```python
from build123d import *

# Parameters (mm, degrees)
BOSS_EXTRUDE1_DEPTH  = 10
M3_CLEARANCE_HOLE1_D = 3.4
FILLET1_R            = 1.5
FILLET2_R            = 0.5


with BuildPart() as part:
    # Sketch1 → Boss-Extrude1 (new body)
    with BuildSketch(Plane.XY):
        with BuildLine():
            ThreePointArc((-5.5, 0), (-5.477033779, -0.502096593), (-5.408326913, -1))
            Line((-5.408326913, -1), (-3.5, -1))
            Line((-3.5, -1), (-3.5, 0))
            ThreePointArc((-3.5, 0), (0, 3.5), (3.5, 0))
            Line((3.5, 0), (3.5, -1))
            Line((3.5, -1), (5.408326913, -1))
            ThreePointArc((5.408326913, -1), (5.477033779, -0.502096593), (5.5, 0))
            ThreePointArc((5.5, 0), (0, 5.5), (-5.5, 0))
        make_face()
        with BuildLine():
            Line((5.5, -1), (5.5, 0))
            ThreePointArc((5.5, 0), (5.477033779, -0.502096593), (5.408326913, -1))
            Line((5.408326913, -1), (5.5, -1))
        make_face()
        with BuildLine():
            Line((-5.5, 0), (-5.5, -1))
            Line((-5.5, -1), (-5.408326913, -1))
            ThreePointArc((-5.408326913, -1), (-5.477033779, -0.502096593), (-5.5, 0))
        make_face()
        with BuildLine():
            Line((-5.5, -1), (-12, -1))
            Line((-12, -1), (-12, -3))
            Line((-12, -3), (-4.609772229, -3))
            ThreePointArc((-4.609772229, -3), (-5.107893656, -2.039466204), (-5.408326913, -1))
            Line((-5.408326913, -1), (-5.5, -1))
        make_face()
        with BuildLine():
            Line((-3.5, -1), (-5.408326913, -1))
            ThreePointArc((-5.408326913, -1), (-5.107893656, -2.039466204), (-4.609772229, -3))
            Line((-4.609772229, -3), (-3.5, -3))
            Line((-3.5, -3), (-3.5, -1))
        make_face()
        with BuildLine():
            Line((3.5, -3), (4.609772229, -3))
            ThreePointArc((4.609772229, -3), (5.107893656, -2.039466204), (5.408326913, -1))
            Line((5.408326913, -1), (3.5, -1))
            Line((3.5, -1), (3.5, -3))
        make_face()
        with BuildLine():
            ThreePointArc((5.408326913, -1), (5.107893656, -2.039466204), (4.609772229, -3))
            Line((4.609772229, -3), (12, -3))
            Line((12, -3), (12, -1))
            Line((12, -1), (5.5, -1))
            Line((5.5, -1), (5.408326913, -1))
        make_face()
    extrude(amount=BOSS_EXTRUDE1_DEPTH)

    # M3 Clearance Hole1 (through all)
    with Locations(Plane(origin=(0, -1, 0), x_dir=(1, 0, 0), z_dir=(0, 1, 0))):
        with Locations((9, -5), (-9, -5)):
            Hole(M3_CLEARANCE_HOLE1_D / 2)

    # Fillet1
    fillet1_edges = [part.edges().sort_by_distance(p)[0] for p in [
        (12, -2, 0),
        (-12, -2, 0),
        (-12, -2, 10),
        (12, -2, 10),
    ]]
    fillet(fillet1_edges, radius=FILLET1_R)

    # Fillet2
    fillet2_edges = [part.edges().sort_by_distance(p)[0] for p in [
        (5.5, -0.5, 10),
        (7, -3, 0),
        (0, 5.5, 10),
        (3.5, -1.5, 0),
        (0, 3.5, 0),
        (-3.5, -1.5, 0),
        (-5.5, -0.5, 0),
        (0, 5.5, 0),
        (5.5, -0.5, 0),
        (-5.5, -0.5, 10),
        (8, -1, 0),
        (3.5, -3, 5),
        (-3.5, -3, 5),
        (-3.5, -1.5, 10),
        (0, 3.5, 10),
        (8, -1, 10),
        (3.5, -1.5, 10),
        (12, -1, 5),
        (12, -3, 5),
        (11.560660172, -3, 0.439339828),
        (11.560660172, -3, 9.560660172),
        (7, -3, 10),
        (-8, -1, 10),
        (-7, -3, 10),
        (11.560660172, -1, 0.439339828),
        (11.560660172, -1, 9.560660172),
        (-7, -3, 0),
        (-8, -1, 0),
        (-12, -3, 5),
        (-12, -1, 5),
        (-11.560660172, -3, 9.560660172),
        (-11.560660172, -3, 0.439339828),
        (-11.560660172, -1, 9.560660172),
        (-11.560660172, -1, 0.439339828),
    ]]
    fillet(fillet2_edges, radius=FILLET2_R)


solid = part.part
```
Input: part model. Units: mm. Frame: model coordinates. A direction names the side the tool comes from. Give positions to 0.01 mm unless a question says otherwise; leave off trailing zeros. Loops run counter-clockwise (first coordinate to the right, second up) from the corner with the lowest first, then second, coordinate; pieces in that order, holes last. Notation, with made-up numbers: M -19,22.5 L 6,22.5 A21 ccw 6,37.5 Z; hole C -11.75,-33 d6. An arc over 180 degrees is marked long. Answer as CSV lines item,"result". Start each with the question number.
1. Section B-B on x = 9. Return loops of the section in (y, z).
2. Section A-A on y = -2.25. Return loops of the section in (x, z), plus the area to 3 significant figures.
3. Section D-D on z = 8. Return loops of the section in (x, y).
4. Pull-direction query (X, two-part tool) for faces 6 (the face through (-5.5, -0.5, 4.9)), 7 (the face through (-0.1, 3.5, 4.9)), 8 (the face through (12, -2, 5)); classes: released by +X, released by -X, zero draft, split by the parting line, or undercut.
5. Reachability of faces 1 (the face through (-2, 4, 10)), 2 (the face through (-7, -1, 5)), 3 (the face through (-11.55, -2.01, 9.57)), 4 (the face through (5.5, -0.5, 4.9)), 5 (the face through (3.5, -1, 5)) from +Z, -Z, +X, -X, +Y, -Y: full face, straight path, thin tool, end or side. Return the list, or none.
6. Pin query (flat end, axial travel): P1, Ø1, axis at x = 3, y = 2, coming from the -Z side; P2, Ø3, axis at y = 2.5, z = 1.5, coming from the +X side; P3, Ø0.5, axis at y = -0.5, z = 3, coming from the +X side; P4, Ø1.8, axis at x = 7, z = 5.5, coming from the +Y side. Return the tip coordinate at first contact, or that it passes through.
7. Section C-C on z = 5. Return loops of the section in (x, y).
8. Line query: L1, parallel to X at y = -2.3, z = 5; L2, parallel to Z at x = 9, y = -1.45; L3, parallel to X at y = 0, z = 4.75. Output: solid intervals per line, ascending.
Computed values:
1,outline,"M -3,0.5 A0.5 ccw -2.5,0 L -1.5,0 A0.5 ccw -1,0.5 L -1,3.3 L -3,3.3 Z; M -3,6.7 L -1,6.7 L -1,9.5 A0.5 ccw -1.5,10 L -2.5,10 A0.5 ccw -3,9.5 Z"
2,outline,"M -12,1.5 A1.5 ccw -10.5,0 L -4,0 A0.5 ccw -3.5,0.5 L -3.5,9.5 A0.5 ccw -4,10 L -10.5,10 A1.5 ccw -12,8.5 Z; M 3.5,0.5 A0.5 ccw 4,0 L 10.5,0 A1.5 ccw 12,1.5 L 12,8.5 A1.5 ccw 10.5,10 L 4,10 A0.5 ccw 3.5,9.5 Z; hole C -9,5 d3.4; hole C 9,5 d3.4"
2,area,"150 mm²"
3,outline,"M -12,-2.5 A0.5 ccw -11.5,-3 L -4,-3 A0.5 ccw -3.5,-2.5 L -3.5,0 A3.5 cw 3.5,0 L 3.5,-2.5 A0.5 ccw 4,-3 L 11.5,-3 A0.5 ccw 12,-2.5 L 12,-1.5 A0.5 ccw 11.5,-1 L 5.5,-1 L 5.5,0 A5.5 ccw -5.5,0 L -5.5,-1 L -11.5,-1 A0.5 ccw -12,-1.5 Z"
4,face 6,"released by -X"
4,face 7,"undercut"
4,face 8,"released by +X"
5,face 1,"+Z, +X, -X, +Y, -Y"
5,face 2,"+Z, -Z, -X, +Y"
5,face 3,"+Z, -X, +Y, -Y"
5,face 4,"+Z, -Z, +X, +Y"
5,face 5,"+Z, -Z, -Y"
6,P1,"stops at z = 0"
6,P2,"stops at x = 5.41"
6,P3,"stops at x = 5.5"
6,P4,"stops at y = -1"
7,outline,"M -12,-2.5 A0.5 ccw -11.5,-3 L -10.7,-3 L -10.7,-1 L -11.5,-1 A0.5 ccw -12,-1.5 Z; M -7.3,-3 L -4,-3 A0.5 ccw -3.5,-2.5 L -3.5,0 A3.5 cw 3.5,0 L 3.5,-2.5 A0.5 ccw 4,-3 L 7.3,-3 L 7.3,-1 L 5.5,-1 L 5.5,0 A5.5 ccw -5.5,0 L -5.5,-1 L -7.3,-1 Z; M 10.7,-3 L 11.5,-3 A0.5 ccw 12,-2.5 L 12,-1.5 A0.5 ccw 11.5,-1 L 10.7,-1 Z"
8,L1,"x = -12 to -10.7, -7.3 to -3.5, 3.5 to 7.3, 10.7 to 12"
8,L2,"z = 0 to 3.3, 6.7 to 10"
8,L3,"x = -5.5 to -3.5, 3.5 to 5.5"
